CAD build for the part. Positions are in the model's coordinates, mm. Face numbers are marked on the shaded views. A direction names the side the tool comes from. Give positions to 0.01 mm unless a question says otherwise; leave off trailing zeros. Order: outer loops, then holes, each group sorted by start corner. A loop starts at its lowest first (then second) coordinate and runs counter-clockwise, first axis right, second up. Notation, with made-up numbers: M -10.75,81 L 22.25,81 A23 ccw 22.25,118 Z; hole C -6,63.5 d2. An arc over 180 degrees is marked long. Put each result on its own line as item: value. Start each with the question number.
1) Cut at A-A (y = -3.5). Write the cut outline in (x, z) (3 decimals).
2) Two-plate mould, pull along X, no slides. Class the marked faces 6, 7 and 8: released by +X, released by -X, zero draft, split by the parting line, or undercut.
3) Pin check, flat tip, straight feed: pin 1 (2.5 mm diameter, centred on y = -5, z = -9, fed in from +X). Stop position of the tip, or through.
4) Tool access for the marked faces 1, 2, 3, 4 and 5: list every direction of +Z, -Z, +X, -X, +Y, -Y with a clear straight run to the whole face (end or side of a thin tool).
5) Cut at D-D (x = -15). Write the cut outline in (y, z) (3 decimals), and give its area (3 significant figures).
6) Drill centre lines: line 1 (X direction, y = -3.45, z = -8.8) (3 decimals); line 2 (Z direction, x = -9, y = -6); line 3 (Z direction, x = -14, y = -4.5). Where is each one in solid material? Low to high. Write a range as [from, to].
7) Cut at B-B (x = 0). Write the cut outline in (y, z) (3 decimals).
8) Cut at C-C (z = -9.5). Write the cut outline in (x, y) (3 decimals), and give its area (3 significant figures).
```python
from build123d import *

# Parameters (mm, degrees)
F2_DEPTH  = 8
F3_W      = 40
F3_H      = 13.08
F4_DEPTH  = 2
F8_DEPTH  = 25.4
F9_DEPTH  = 0.2869853
F10_DEPTH = 0.2869852618
F11_DEPTH = 1.225
F13_DEPTH = 25.4


# Not quite as in the source:
# - an extrude ends at something that could not be found from the text; its depth is read off the source's solid


with BuildPart() as f2:
    # F1 (on Front) → F2 (new body)
    with BuildSketch(Plane.XZ):
        with BuildLine():
            Line((0, -2.26), (-20, -2.26))
            Line((-20, -2.26), (-20, -4.8))
            Line((-20, -4.8), (-7.175, -4.8))
            ThreePointArc((-7.175, -4.8), (-3.3907124319, -10.0958269953), (-9.6268909943, -11.9604161992))
            Line((-9.6268909943, -11.9604161992), (-15.6340319663, -7.3))
            Line((-15.6340319663, -7.3), (-20, -7.3))
            Line((-20, -7.3), (-20, -15.34))
            Line((-20, -15.34), (0, -15.34))
            Line((0, -15.34), (20, -15.34))
            Line((20, -15.34), (20, -7.3))
            Line((20, -7.3), (15.6340319663, -7.3))
            Line((15.6340319663, -7.3), (9.6268909943, -11.9604161992))
            ThreePointArc((9.6268909943, -11.9604161992), (3.3907124319, -10.0958269953), (7.175, -4.8))
            Line((7.175, -4.8), (20, -4.8))
            Line((20, -4.8), (20, -2.26))
            Line((20, -2.26), (0, -2.26))
        make_face()
    extrude(amount=F2_DEPTH)


with BuildPart() as f2b:
    # F1 (on Front) → F2, piece 2 (new body)
    with BuildSketch(Plane.XZ):
        with BuildLine():
            Line((-14.4153116271, -6.3), (-8.7175368467, -10.7673789865))
            ThreePointArc((-8.7175368467, -10.7673789865), (-4.8119037825, -9.6159511424), (-7.175, -6.3))
            Line((-7.175, -6.3), (-14.4153116271, -6.3))
        make_face()
    extrude(amount=F2_DEPTH)


with BuildPart() as f2c:
    # F1 (on Front) → F2, piece 3 (new body)
    with BuildSketch(Plane.XZ):
        with BuildLine():
            Line((8.7175368467, -10.7673789865), (14.4153116271, -6.3))
            Line((14.4153116271, -6.3), (7.175, -6.3))
            ThreePointArc((7.175, -6.3), (4.8119037825, -9.6159511424), (8.7175368467, -10.7673789865))
        make_face()
    extrude(amount=F2_DEPTH)


with BuildPart() as f4:
    # F3 (on face) → F4 (new body)
    with BuildSketch(Plane(origin=(0, 0, 0), x_dir=(-1, 0, 0), z_dir=(0, 1, 0))):
        with Locations((0, -8.8)):
            Rectangle(F3_W, F3_H)
    extrude(amount=-F4_DEPTH)

    # F5: union F2
    add(f2.part)


with BuildPart() as f2c_1:
    add(f2c.part)

    # F6: union F4, F2b
    add(f4.part)
    add(f2b.part)

    # F7 (on face) → F8 (cut)
    with BuildSketch(Plane.XZ.offset(8)):
        with BuildLine():
            Line((22.5005224347, -7.3), (20, -7.3))
            Line((20, -7.3), (19.7130147382, -7.3))
            Line((19.7130147382, -7.3), (11.7279629554, -13.4949045067))
            ThreePointArc((11.7279629554, -13.4949045067), (9.6313107017, -14.8611993646), (7.175, -15.34))
            Line((7.175, -15.34), (7.175, -19.2080270499))
            Line((7.175, -19.2080270499), (22.5005224347, -19.2080270499))
            Line((22.5005224347, -19.2080270499), (22.5005224347, -7.3))
        make_face()
        with BuildLine():
            Line((-19.7130147382, -7.3), (-20, -7.3))
            Line((-20, -7.3), (-22.5005224347, -7.3))
            Line((-22.5005224347, -7.3), (-22.5005224347, -19.2080270499))
            Line((-22.5005224347, -19.2080270499), (-7.175, -19.2080270499))
            Line((-7.175, -19.2080270499), (-7.175, -15.34))
            ThreePointArc((-7.175, -15.34), (-9.6313107017, -14.8611993646), (-11.7279629554, -13.4949045067))
            Line((-11.7279629554, -13.4949045067), (-19.7130147382, -7.3))
        make_face()
    extrude(amount=-F8_DEPTH, mode=Mode.SUBTRACT)

    # F9 (cut, through all): a face of the model
    f9_faces = [f2c_1.faces().sort_by_distance(p)[0] for p in [
        (20, -3.4075829384, -4.0276303318),
    ]]
    extrude(f9_faces, amount=-F9_DEPTH, mode=Mode.SUBTRACT)

    # F10 (cut, through all): a face of the model
    f10_faces = [f2c_1.faces().sort_by_distance(p)[0] for p in [
        (-20, -3.4075829384, -4.0276303318),
    ]]
    extrude(f10_faces, amount=-F10_DEPTH, mode=Mode.SUBTRACT)

    # F11 (add): a face of the model
    f11_faces = [f2c_1.faces().sort_by_distance(p)[0] for p in [
        (-8.8e-09, 0, -8.042025569),
    ]]
    extrude(f11_faces, amount=F11_DEPTH)

    # F12 (on face) → F13 (cut)
    with BuildSketch(Plane.XZ.offset(8)):
        with BuildLine():
            ThreePointArc((-1.5, -11.34), (0, -12.84), (1.5, -11.34))
            Line((1.5, -11.34), (1.5, -6.26))
            ThreePointArc((1.5, -6.26), (0, -4.76), (-1.5, -6.26))
            Line((-1.5, -6.26), (-1.5, -11.34))
        make_face()
    extrude(amount=-F13_DEPTH, mode=Mode.SUBTRACT)


solid = f2c_1.part
```
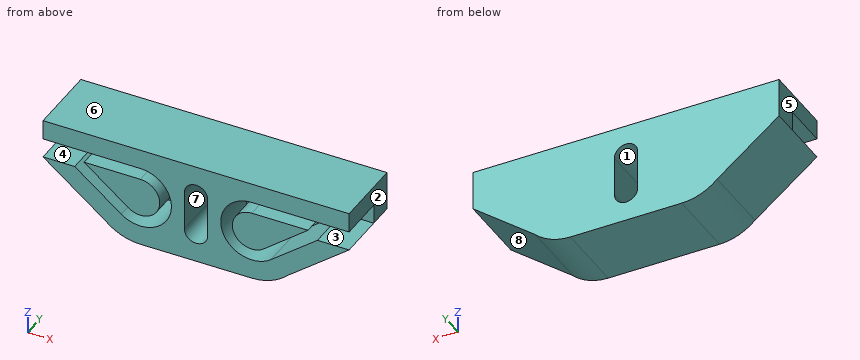
Solution:
1. outline: M -19.713,-7.3 L -11.728,-13.495 A6.54 ccw -7.175,-15.34 L 7.175,-15.34 A6.54 ccw 11.728,-13.495 L 19.713,-7.3 L 15.634,-7.3 L 9.627,-11.96 A4 cw long 7.175,-4.8 L 19.713,-4.8 L 19.713,-2.26 L -19.713,-2.26 L -19.713,-4.8 L -7.175,-4.8 A4 cw long -9.627,-11.96 L -15.634,-7.3 Z; M -14.415,-6.3 L -8.718,-10.767 A2.5 ccw long -7.175,-6.3 Z; M 7.175,-6.3 A2.5 ccw long 8.718,-10.767 L 14.415,-6.3 Z; hole M -1.5,-11.34 A1.5 ccw 1.5,-11.34 L 1.5,-6.26 A1.5 ccw -1.5,-6.26 Z
2. face 6: zero draft
2. face 7: undercut
2. face 8: released by +X
3. pin 1: x = 19.13
4. face 1: +Y, -Y
4. face 2: +Z, -Z, +X, +Y, -Y
4. face 3: +X, -Y
4. face 4: -X, -Y
4. face 5: +Z, -Z, -X, +Y, -Y
5. outline: M -8,-10.956 L 1.225,-10.956 L 1.225,-2.26 L -8,-2.26 L -8,-4.8 L -2,-4.8 L -2,-7.792 L -8,-7.792 Z
5. area: 62.3 mm²
6. line 1: [-17.78, -13.701], [-11.227, -4.675], [-3.175, -1.5], [1.5, 3.175], [4.675, 11.227], [13.701, 17.78]
6. line 2: [-15.08, -12.36], [-10.55, -6.3], [-4.8, -2.26]
6. line 3: [-11.73, -8.57], [-6.63, -6.3], [-4.8, -2.26]
7. outline: M -8,-15.34 L 1.225,-15.34 L 1.225,-12.84 L -8,-12.84 Z; M -8,-4.76 L 1.225,-4.76 L 1.225,-2.26 L -8,-2.26 Z
8. outline: M -16.877,-8 L -12.798,-8 L -12.798,-2 L -10.334,-2 L -10.334,-8 L -4.775,-8 L -4.775,-2 L -3.237,-2 L -3.237,-8 L -1.5,-8 L -1.5,1.225 L -16.877,1.225 Z; M 1.5,-8 L 3.237,-8 L 3.237,-2 L 4.775,-2 L 4.775,-8 L 10.334,-8 L 10.334,-2 L 12.798,-2 L 12.798,-8 L 16.877,-8 L 16.877,1.225 L 1.5,1.225 Z
8. area: 236 mm²
